```python
from build123d import *

# Parameters (mm, degrees)
F0_R     = 13.95
F1_DEPTH = 16.1
F2_R     = 2.5
F3_DEPTH = 15
F4_R     = 1.5
F5_DEPTH = 4
F6_R     = 2


with BuildPart() as f1:
    # F0 (on Front) → F1 (new body)
    with BuildSketch(Plane.XZ):
        Circle(F0_R)
    extrude(amount=-F1_DEPTH)

    # F2 (on face) → F3 (join)
    with BuildSketch(Plane(origin=(0, 16.1, 0), x_dir=(-1, 0, 0), z_dir=(0, 1, 0))):
        Circle(F2_R)
    extrude(amount=F3_DEPTH)

    # F4 (on face) → F5 (cut)
    with BuildSketch(Plane.XZ):
        with Locations((0, 9.5)):
            Circle(F4_R)
        with Locations((0, -9.5)):
            Circle(F4_R)
        with Locations((-8, 0)):
            Circle(F4_R)
        with Locations((8, 0)):
            Circle(F4_R)
    extrude(amount=-F5_DEPTH, mode=Mode.SUBTRACT)

    # F6
    f6_edges = [f1.edges().sort_by_distance(p)[0] for p in [
        (13.95, 8.05, 0),
        (-13.95, 0, 0),
        (-13.95, 16.1, 0),
    ]]
    fillet(f6_edges, radius=F6_R)


solid = f1.part
```
Work out the finished part from the listing and answer in its coordinate system (mm). A direction names the side the tool comes from. Coordinates: 2 decimals unless noted, no trailing zeros. Write each loop counter-clockwise with the first axis right and the second up, starting at its lowest first coordinate (ties: lowest second). Pieces come first, ordered by that corner, then holes.
Q1. Which of the six approach directions +Z, -Z, +X, -X, +Y, -Y give full straight-line access (tool end or side, diameter ignored) to faces 4 (the face through (0, 0, 0)), 5 (the face through (0.54, 23.5, -2.44)), 6 (the face through (-9.5, 1.97, 0.07))?
Q2. A cutting plane is placed at B-B, the plane x = 0. Give the vertices of the cut face in (y, z), then the cut area to 3 significant figures.
Q3. Each of these flat-tipped pins is pushed along its axis until it touches: pin 1 Ø0.9 at (x, z) = (7.5, 0) entering from -Y; pin 2 Ø2.5 at (x, z) = (8, 0) entering from +Y; pin 3 Ø1 at (x, y) = (-5, 4) entering from +Z. Where does it stop, or does it pass through?
Q4. A cutting plane is placed at A-A, the plane z = 0. Give the vertices of the cut face in (x, y), then the cut area to 3 significant figures.
Q5. A cutting plane is placed at D-D, the plane y = 28. Give the vertices of the cut face in (x, z).
Q6. Find the intervals of material crossed by line 1 (Y direction, x = 0.75, z = -5.5); line 2 (Z direction, x = -0.75, y = 2); line 3 (Y direction, x = 0.25, z = -8.25), in increasing order.
Q7. A cutting plane is placed at C-C, the plane y = 6. Give the vertices of the cut face in (x, z).
Q8. Determine the mould class of faces 1 (the face through (-3.02, 7.97, -13.62)), 2 (the face through (0, 4, -9)), 3 (the face through (0, 31.1, 0)) for opening direction X: released by +X, released by -X, zero draft, split by the parting line, or undercut.
Findings below:
1. face 4: +Z, -Z, +X, -X, -Y
1. face 5: +Y
1. face 6: -Y
2. outline: (0, -11.95) arc R2 ccw to (2, -13.95) - (14.1, -13.95) arc R2 ccw to (16.1, -11.95) - (16.1, -2.5) - (31.1, -2.5) - (31.1, 2.5) - (16.1, 2.5) - (16.1, 11.95) arc R2 ccw to (14.1, 13.95) - (2, 13.95) arc R2 ccw to (0, 11.95) - (0, 11) - (4, 11) - (4, 8) - (0, 8) - (0, -8) - (4, -8) - (4, -11) - (0, -11) - close
2. area: 497 mm2
3. pin 1: stops at y = 4
3. pin 2: stops at y = 16.1
3. pin 3: stops at z = 13.2
4. outline: (-13.95, 2) arc R2 ccw to (-11.95, 0) - (-9.5, 0) - (-9.5, 4) - (-6.5, 4) - (-6.5, 0) - (6.5, 0) - (6.5, 4) - (9.5, 4) - (9.5, 0) - (11.95, 0) arc R2 ccw to (13.95, 2) - (13.95, 14.1) arc R2 ccw to (11.95, 16.1) - (2.5, 16.1) - (2.5, 31.1) - (-2.5, 31.1) - (-2.5, 16.1) - (-11.95, 16.1) arc R2 ccw to (-13.95, 14.1) - close
4. area: 497 mm2
5. outline: circle Ø5 at (0, 0)
6. line 1: y = 0 to 16.1
6. line 2: z = -13.93 to -10.8, -8.2 to 8.2, 10.8 to 13.93
6. line 3: y = 4 to 16.1
7. outline: circle Ø27.9 at (0, 0)
8. face 1: split by the parting line
8. face 2: undercut
8. face 3: zero draft
